Part model, mm, in its own coordinate system. A direction names the side the tool comes from. Round coordinates to 2 decimals unless told otherwise and drop trailing zeros. Loops run counter-clockwise (first coordinate to the right, second up) from the corner with the lowest first, then second, coordinate; pieces in that order, holes last.
1) 3-axis set-ups, long thin cutter, end or side, ignore diameter. For faces 1 (the flat face through (1.33, 3, -3)), 2 (the flat face through (2, 3, -3.627)): which of +Z, -Z, +X, -X, +Y, -Y reach the whole face in a straight line?
2) Band-saw the part on B-B, the plane y = 5.15. Write the cut outline in (x, z), then the cut area to 3 significant figures.
3) Probe line 1 (X direction, y = 3.45, z = 0); line 2 (X direction, y = 1.8, z = -3); line 3 (Z direction, x = 0, y = 1.95). List the from-to ranges inside material, lowest first.
4) Band-saw the part on D-D, the plane x = 0. Write the cut outline in (y, z), then the cut area to 3 significant figures.
5) Band-saw the part on C-C, the plane z = 2. Write the cut outline in (x, y).
6) Drop a flat-ended pin along its axis: P1, Ø1.5, axis at x = 0, y = 0.5, coming from the -Z side. Give the stop position or say it passes through.
7) Band-saw the part on A-A, the plane z = 0. Write the cut outline in (x, y), then the cut area to 3 significant figures.
8) Mould opens along X. For faces 3 (the cylindrical face through (-0.08, 2.96, 2.25)), 4 (the flat face through (3, 3, 0)), 5 (the flat face through (-1.33, 3, -3)), 6 (the flat face through (-2, 3, -3.627)) say: +X half, -X half, draft (parallel to the pull), parting line (faces both ways), or undercut.
from build123d import *

# Parameters (mm, degrees)
EXTRUDE_1_DEPTH = 6


with BuildPart() as part:
    # Эскиз1 → Бобышка-Вытянуть1 (new body)
    with BuildSketch(Plane(origin=(0, 0, 0), x_dir=(1, 0, 0), z_dir=(0, 1, 0))):
        with BuildLine():
            Line((-3, 3.627046628), (-1.330273321, 3.627046628))
            Line((-1.330273321, 3.627046628), (-1.330273321, 1.81462748))
            ThreePointArc((-1.330273321, 1.81462748), (0, -2.25), (1.330273321, 1.81462748))
            Line((1.330273321, 1.81462748), (1.330273321, 3.627046628))
            Line((1.330273321, 3.627046628), (3, 3.627046628))
            Line((3, 3.627046628), (3, -3.627046628))
            Line((3, -3.627046628), (-3, -3.627046628))
            Line((-3, -3.627046628), (-3, 3.627046628))
        make_face()
    extrude(amount=EXTRUDE_1_DEPTH)


solid = part.part
Reported:
1. face 1: -Z, +Y, -Y
1. face 2: -Z, +X, -X, +Y, -Y
2. outline: (-3, -3.63) - (-1.33, -3.63) - (-1.33, -1.81) arc R2.25 cw (long way) to (1.33, -1.81) - (1.33, -3.63) - (3, -3.63) - (3, 3.63) - (-3, 3.63) - close
2. area: 23.6 mm2
3. line 1: x = -3 to -2.25, 2.25 to 3
3. line 2: x = -3 to -1.33, 1.33 to 3
3. line 3: z = 2.25 to 3.63
4. outline: (0, 2.25) - (6, 2.25) - (6, 3.63) - (0, 3.63) - close
4. area: 8.26 mm2
5. outline: (-3, 0) - (-1.03, 0) - (-1.03, 6) - (-3, 6) - close; (1.03, 0) - (3, 0) - (3, 6) - (1.03, 6) - close
6. P1: stops at z = 2.12
7. outline: (-3, 0) - (-2.25, 0) - (-2.25, 6) - (-3, 6) - close; (2.25, 0) - (3, 0) - (3, 6) - (2.25, 6) - close
7. area: 9.00 mm2
8. face 3: undercut
8. face 4: +X half
8. face 5: undercut
8. face 6: draft
